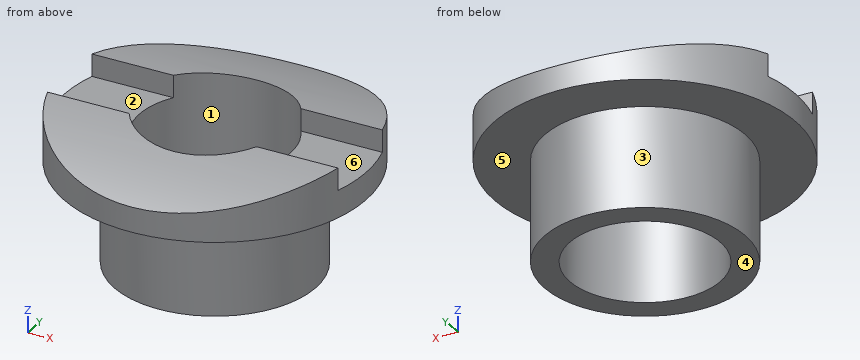
```python
from build123d import *

# Parameters (mm, degrees)
SKETCH1_R               = 3.175
SKETCH1_R_2             = 2.38125
BOSS_EXTRUDE1_DEPTH     = 3.175
SKETCH2_R               = 4.7625
SKETCH2_R_2             = 2.38125
BOSS_EXTRUDE2_DEPTH     = 1.6256
SKETCH3_R               = 22.361166229
SKETCH3_R_2             = 13.97
CUT_EXTRUDE1_DEPTH      = 5.7625
CUT_EXTRUDE1_DEPTH_BACK = 5.7625
SKETCH4_W               = 0.762
SKETCH4_H               = 2.54
CUT_EXTRUDE2_DEPTH      = 5.7625001
CUT_EXTRUDE2_DEPTH_BACK = 5.7625001


with BuildPart() as part:
    # Sketch1 → Boss-Extrude1 (new body)
    with BuildSketch(Plane.XY):
        Circle(SKETCH1_R)
        Circle(SKETCH1_R_2, mode=Mode.SUBTRACT)
    extrude(amount=BOSS_EXTRUDE1_DEPTH)

    # Sketch2 → Boss-Extrude2 (add)
    with BuildSketch(Plane.XY.offset(3.175)):
        Circle(SKETCH2_R)
        Circle(SKETCH2_R_2, mode=Mode.SUBTRACT)
    extrude(amount=BOSS_EXTRUDE2_DEPTH)

    # Sketch3 → Cut-Extrude1 (cut, two sides)
    with BuildSketch(Plane(origin=(0, 0, 0), x_dir=(0, 0, -1), z_dir=(1, 0, 0))) as cut_extrude1_sk:
        with Locations((9.1694, 0)):
            Circle(SKETCH3_R)
        with Locations((9.1694, 0)):
            Circle(SKETCH3_R_2, mode=Mode.SUBTRACT)
    extrude(amount=CUT_EXTRUDE1_DEPTH, mode=Mode.SUBTRACT)
    extrude(cut_extrude1_sk.sketch, amount=-CUT_EXTRUDE1_DEPTH_BACK, mode=Mode.SUBTRACT)

    # Sketch4 → Cut-Extrude2 (cut, two sides)
    with BuildSketch(Plane(origin=(0, 0, 0), x_dir=(0, 0, -1), z_dir=(1, 0, 0))) as cut_extrude2_sk:
        with Locations((-4.4196, 0)):
            Rectangle(SKETCH4_W, SKETCH4_H)
    extrude(amount=CUT_EXTRUDE2_DEPTH, mode=Mode.SUBTRACT)
    extrude(cut_extrude2_sk.sketch, amount=-CUT_EXTRUDE2_DEPTH_BACK, mode=Mode.SUBTRACT)


solid = part.part
```
Part model, mm, in its own coordinate system. Face numbers are marked on the shaded views. A direction names the side the tool comes from. Coordinates: 2 decimals unless noted, no trailing zeros. Order: outer loops, then holes, each group sorted by start corner. A loop starts at its lowest first (then second) coordinate and runs counter-clockwise, first axis right, second up. Notation, with made-up numbers: (31.25, -35) - (85.25, -35) arc R26 ccw to (85.25, -17) - close; hole circle Ø6 at (72.25, 58.5). An arc over 180 degrees is marked (long way). Return JSON: item names as keys, results as strings. Group by question number.
Item 1: Cut at A-A (y = 0). List the corners of the cut face in (x, z) (1 decimal).
Item 2: Which spindle directions (+Z, -Z, +X, -X, +Y, -Y) get a long thin tool onto all of the face, cutting with end or side? Do the marked faces 4, 5 and 6. Say none if no direction does.
Item 3: Pull direction X, two halves, no side cores. Call the marked faces 1, 2 and 3: pulls with the +X half, pulls with the -X half, needs draft (parallel to the pull), parting line crosses it, or undercut.
Item 4: Cut at D-D (x = 3). List the corners of the cut face in (y, z) (3 decimals), plus the area to 3 significant figures.
Item 5: Cut at B-B (x = -1.5). List the corners of the cut face in (y, z) (3 decimals).
Item 6: Drill centre lines: probe 1 along Y at (x, z) = (0, 3.7); probe 2 along Y at (x, z) = (0, 1.75) (3 decimals); probe 3 along X at (y, z) = (2, 1.05). Where is each one in solid material? Low to high. Write a range as from..to.
Item 7: Cut at C-C (z = 3.6). List the corners of the cut face in (x, y) (1 decimal).
Item 8: Pin check, flat tips, straight feed: pin 1 (1.5 mm diameter, centred on y = -2.5, z = 2, fed in from -X); pin 2 (2 mm diameter, centred on x = -3, y = 0, fed in from +Z); pin 3 (5 mm diameter, centred on x = 0, y = -2, fed in from -Z); pin 4 (0.8 mm diameter, centred on x = 3, z = 4.5, fed in from -Y). Stop position of each tip, or through.
Check values:
{
 "1": {"outline": "(-4.8, 3.2) - (-3.2, 3.2) - (-3.2, 0) - (-2.4, 0) - (-2.4, 4) - (-4.8, 4) - close; (2.4, 0) - (3.2, 0) - (3.2, 3.2) - (4.8, 3.2) - (4.8, 4) - (2.4, 4) - close"},
 "2": {"face 4": "-Z, +X, -X, +Y, -Y", "face 5": "-Z", "face 6": "+Z, +X, -X"},
 "3": {"face 1": "undercut", "face 2": "needs draft", "face 3": "parting line crosses it"},
 "4": {"outline": "(-3.699, 3.175) - (-1.04, 3.175) - (-1.04, 0) - (1.04, 0) - (1.04, 3.175) - (3.699, 3.175) - (3.699, 4.302) arc R13.97 ccw to (1.27, 4.743) - (1.27, 4.039) - (-1.27, 4.039) - (-1.27, 4.743) arc R13.97 ccw to (-3.699, 4.302) - close", "area": "15.5 mm2"},
 "5": {"outline": "(-4.52, 3.175) - (-2.798, 3.175) - (-2.798, 0) - (-1.849, 0) - (-1.849, 4.678) arc R13.97 ccw to (-4.52, 4.049) - close; (1.849, 0) - (2.798, 0) - (2.798, 3.175) - (4.52, 3.175) - (4.52, 4.049) arc R13.97 ccw to (1.849, 4.678) - close"},
 "6": {"probe 1": "y = -4.76..-2.38, 2.38..4.76", "probe 2": "y = -3.175..-2.381, 2.381..3.175", "probe 3": "x = -2.47..-1.29, 1.29..2.47"},
 "7": {"outline": "circle Ø9.5 at (0, 0); hole circle Ø4.8 at (0, 0)"},
 "8": {"pin 1": "stops at x = -2.65", "pin 2": "stops at z = 4.04", "pin 3": "stops at z = 0", "pin 4": "stops at y = -3.92"}
}
